Geometry: final body of the model. Coordinates: model frame, mm. Face numbers are marked on the shaded views. A direction names the side the tool comes from. Give positions to 0.01 mm unless a question says otherwise; leave off trailing zeros. Loops run counter-clockwise (first coordinate to the right, second up) from the corner with the lowest first, then second, coordinate; pieces in that order, holes last. Notation, with made-up numbers: (-9, 43.5) -> (42, 43.5) arc R23 ccw to (42, 74.5) -> close; hole circle Ø3 at (71, 87.25). An arc over 180 degrees is marked (long way). Answer in a Markdown table with one row per item. Add a question column.
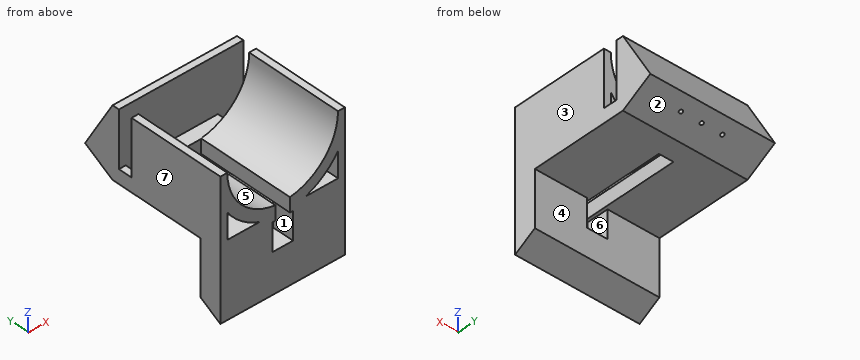
Autodesk Inventor part; units mm, degrees
ref_plane "YZ Plane" through (0, 0, 0) normal (1, 0, 0) x (0, 1, 0)
ref_plane "XZ Plane" through (0, 0, 0) normal (0, 1, 0) x (-1, 0, 0)
ref_plane "XY Plane" through (0, 0, 0) normal (0, 0, 1) x (1, 0, 0)
sketch "スケッチ1" plane through (0, 0, 0) normal (0, 1, 0) x (-1, 0, 0)
  line L0 (0, 0) -> (-90, 0)
  line L1 (-90, 0) -> (-90, 50)
  line L2 (0, 50) -> (0, 0)
  line L3 (0, 0) -> (-5, 0)
  line L4 (-5, 0) -> (-5, 50)
  line L5 (-5, 0) -> (-90, 0)
  line L6 (-90, 0) -> (-85, 0)
  line L7 (-85, 0) -> (-85, 50)
  arc A0 (-85, 50) -> (-5, 50) centre (-45, 50) ccw
  line L8 (0, 0) -> (0, 10)
  line L9 (0, 10) -> (-90, 10)
  circle A1 centre (-45, 50) radius 45
  line L10 (-90, 5) -> (0, 5)
  line L11 (-90, 50) -> (-85, 50)
  line L12 (-5, 50) -> (0, 50)
  line L13 (0, 0) -> (-90, 0)
  line L14 (-90, 0) -> (-90, 5)
  line L15 (-90, 5) -> (0, 5)
  line L16 (0, 5) -> (0, 0)
  dimension "d0" = 90
  dimension "d1" = 50
  dimension "d2" = 5
  dimension "d3" = 85
  dimension "d4" = 5
  dimension "d5" = 80
  dimension "d6" = 10
  dimension "d7" = 90
extrude "押し出し1" add sketch "スケッチ1" along normal blind 230 contours L0 L4 L10 L2 | L0 L7 L10 L4 | L10 L4 L9 L2 | L0 L1 L10 L7 | L10 A1 L9 L4 | L9 L4 A1 L2 | L10 L1 L9 L7 | L7 L9 A1 L10 | L9 A1 L4 | A1 L9 | A1 L4 L12 | L9 L1 A1 L7 | L7 A1 L9 | A1 L9 A0 L4 | A1 L7 A0 L9 | L11 L7 A1
sketch "スケッチ2" plane through (0, 0, 0) normal (0, -1, 0) x (1, 0, 0)
  line L0 (0, 0) -> (0, 50)
  line L1 (90, 0) -> (0, 0)
  line L2 (90, 50) -> (90, 0)
  line L3 (85, 50) -> (90, 50)
  arc A0 (5, 50) -> (85, 50) centre (45, 50) ccw
  line L4 (0, 50) -> (5, 50)
  arc A1 (5, 23.467) -> (85, 23.467) centre (45, 50) ccw
  line L5 (0, 5) -> (90, 5)
  line L6 (5, 23.467) -> (5, 5)
  line L7 (85, 23.467) -> (85, 5)
  dimension "d29" = 48
extrude "押し出し2" cut sketch "スケッチ2" against normal blind 225 contours L6 A1 L5 | L5 A1 L7
sketch "スケッチ3" plane through (0, 230, 0) normal (0, 1, 0) x (1, 0, 0)
  arc A0 (85, -50) -> (5, -50) centre (45, -50) ccw
  line L0 (90, -50) -> (90, 0)
  line L1 (0, -50) -> (5, -50)
  arc A1 (85, -50) -> (5, -50) centre (45, -50) ccw
  line L2 (5, -50) -> (85, -50)
extrude "押し出し3" add sketch "スケッチ3" against normal blind 5
sketch "スケッチ4" plane through (90, 0, 50) normal (1, 0, 0) x (0, 0, -1)
  line L0 (0, 0) -> (50, 0)
  line L1 (0, 0) -> (0, 230)
  line L2 (25, 0) -> (25, 65)
  line L3 (25, 65) -> (25, 75)
  line L4 (25, 75) -> (25, 215)
  line L5 (25, 215) -> (25, 225)
  line L6 (0, 65) -> (40, 65)
  line L7 (40, 65) -> (40, 75)
  line L8 (40, 75) -> (0, 75)
  line L9 (0, 75) -> (0, 65)
  line L10 (0, 215) -> (40, 215)
  line L11 (40, 215) -> (40, 225)
  line L12 (40, 225) -> (0, 225)
  line L13 (0, 225) -> (0, 215)
  dimension "d16" = 65
  dimension "d17" = 10
  dimension "d18" = 140
  dimension "d19" = 10
  dimension "d20" = 40
extrude "押し出し4" cut sketch "スケッチ4" against normal blind 90 contours L1 L8 L3 L6 | L3 L8 L7 L6 | L1 L12 L5 L10 | L5 L12 L11 L10
sketch "スケッチ6" plane through (90, 0, 50) normal (1, 0, 0) x (0, 0, -1)
  line L0 (0, 230) -> (50, 230)
  line L1 (50, 230) -> (37.5, 251.6506)
  line L2 (50, 230) -> (110, 230) construction
  line L3 (0, 230) -> (37.5, 251.6506)
  line L4 (0, 230) -> (43.3013, 230) construction
  dimension "d32" = 120
  dimension "d33" = 30
extrude "押し出し6" add sketch "スケッチ6" against normal blind 90
sketch "スケッチ9" plane through (0, 0, 0) normal (-1, 0, 0) x (0, 0, 1)
  line L0 (10, 225) -> (50, 225)
  line L1 (50, 225) -> (50, 230)
  line L2 (50, 230) -> (12.5, 251.6506)
  line L3 (12.5, 251.6506) -> (0, 230)
  line L4 (0, 0) -> (0, 230)
  line L5 (0, 0) -> (50, 0)
  line L6 (50, 0) -> (50, 65)
  line L7 (50, 65) -> (10, 65)
  line L8 (10, 65) -> (10, 75)
  line L9 (10, 75) -> (50, 75)
  line L10 (50, 75) -> (50, 215)
  line L11 (50, 215) -> (10, 215)
  line L12 (10, 215) -> (10, 225)
  line L13 (12.5, 251.6506) -> (0, 230)
  line L14 (0, 230) -> (-132.7906, 0)
  line L15 (0, 145) -> (-49.0748, 145)
  line L16 (0, 115) -> (-66.3953, 115)
  dimension "d45" = 30
sketch "スケッチ10" plane through (0, 0, 0) normal (-1, 0, 0) x (0, 0, 1)
  line L0 (10, 225) -> (50, 225)
  line L1 (50, 225) -> (50, 230)
  line L2 (50, 230) -> (12.5, 251.6506)
  line L3 (12.5, 251.6506) -> (0, 230)
  line L4 (0, 0) -> (0, 230)
  line L5 (0, 0) -> (50, 0)
  line L6 (50, 0) -> (50, 65)
  line L7 (50, 65) -> (10, 65)
  line L8 (10, 65) -> (10, 75)
  line L9 (10, 75) -> (50, 75)
  line L10 (50, 75) -> (50, 215)
  line L11 (50, 215) -> (10, 215)
  line L12 (10, 215) -> (10, 225)
  line L13 (12.5, 251.6506) -> (-87.5, 78.4456)
  line L14 (-87.5, 78.4456) -> (50, 0)
sketch "スケッチ11" plane through (90, 230, 0) normal (0, 0.5, -0.866) x (-1, 0, 0)
  line L0 (0, 25) -> (90, 25)
  line L1 (45, 25) -> (45, 15)
  line L2 (45, 15) -> (60, 15)
  line L3 (60, 15) -> (30, 15)
  point P0 (90, -199.1858)
  dimension "d49" = 10
  dimension "d50" = 15
  dimension "d51" = 30
hole "穴1" at (45, 242.9904, 7.5) at (30, 242.9904, 7.5) at (60, 242.9904, 7.5) direction (0, -0.5, 0.866) diameter 2.5 depth 8 tip angle 118
sketch "スケッチ18" plane through (90, 65, 10) normal (0, 0, 1) x (1, 0, 0)
  line L0 (0, 10) -> (-5, 10)
  line L1 (0, 10) -> (-90, 10)
  line L2 (-90, 10) -> (-90, 150)
  line L3 (-90, 150) -> (0, 150)
  line L4 (0, 150) -> (0, 10)
  line L5 (-45, 150) -> (-45, 10)
  line L6 (-53.1517, 150) -> (-27.646, 150)
  line L7 (-27.646, 150) -> (-27.646, 10)
  line L8 (-27.646, 10) -> (-53.1517, 10)
  line L9 (-53.1517, 10) -> (-53.1517, 150)
  line L10 (-45, 10) -> (-39.75, 10)
  line L11 (-45, 150) -> (-50.25, 150)
  line L12 (-50.25, 150) -> (-39.75, 150)
  line L13 (-39.75, 150) -> (-39.75, 10)
  line L14 (-39.75, 10) -> (-50.25, 10)
  line L15 (-50.25, 10) -> (-50.25, 150)
  point P0 (-90, -65)
  dimension "d76" = 140
  dimension "d77" = 5.25
  dimension "d78" = 5.25
extrude "押し出し12" cut sketch "スケッチ18" against normal blind 10 and the other way blind 5 contours L1 L5 L3 L13 | L1 L15 L3 L5
sketch "スケッチ19" plane through (0, 0, 0) normal (-1, 0, 0) x (0, 0, 1)
  line L0 (10, 225) -> (50, 225)
  line L1 (50, 225) -> (50, 230)
  line L2 (50, 230) -> (12.5, 251.6506)
  line L3 (12.5, 251.6506) -> (0, 230)
  line L4 (0, 0) -> (0, 230)
  line L5 (0, 0) -> (50, 0)
  line L6 (50, 0) -> (50, 65)
  line L7 (50, 65) -> (10, 65)
  line L8 (10, 65) -> (10, 75)
  line L9 (10, 75) -> (50, 75)
  line L10 (50, 75) -> (50, 215)
  line L11 (50, 215) -> (10, 215)
  line L12 (10, 215) -> (10, 225)
  line L13 (0, 230) -> (-23.825, 188.7339)
  line L14 (-23.825, 188.7339) -> (-3.4734, 176.9839)
  circle A0 centre (-3.4734, 176.9839) radius 16
  circle A1 centre (-3.4734, 176.9839) radius 3
  dimension "d83" = 47.65
  dimension "d84" = 23.5
  dimension "d85" = 32
  dimension "d86" = 6
sketch "スケッチ20" plane through (90, 230, 0) normal (0, 0.5, -0.866) x (-1, 0, 0)
  circle A0 centre (60, 15) radius 1.25
  circle A1 centre (45, 15) radius 1.25
  circle A2 centre (30, 15) radius 1.25
  line L0 (0, 0) -> (0, 25)
  line L1 (0, 0) -> (90, 0)
  line L2 (90, 25) -> (90, 0)
  line L3 (0, 25) -> (90, 25)
  point P0 (90, -199.1858)
ref_plane "作業平面5" through (90, 45, 50) normal (0, 1, 0) x (1, 0, 0)
sketch "スケッチ21" plane through (90, 45, 50) normal (0, 1, 0) x (1, 0, 0)
  line L0 (0, 0) -> (-101.8599, 0)
  line L1 (-101.8599, 0) -> (-101.8599, 60.1995)
  line L2 (-101.8599, 60.1995) -> (0, 60.1995)
  line L3 (0, 60.1995) -> (0, 0)
  point P0 (-90, 50)
extrude "押し出し13" cut sketch "スケッチ21" against normal blind 50
ref_plane "作業平面6" through (85, 145, 23.467) normal (0, 1, 0) x (-1, 0, 0)
sketch "スケッチ22" plane through (0, 75, 50) normal (-1, 0, 0) x (0, 0, 1)
  line L0 (-37.5, 176.6506) -> (-50, 155)
  line L1 (-50, -30) -> (-50, 155)
  line L2 (-98.8395, 70.6051) -> (-50, 70.6051)
  line L3 (-107.0544, 55.6051) -> (-50, 55.6051)
  line L4 (-89.7339, 85.6051) -> (-50, 85.6051)
  line L5 (-89.7339, 85.6051) -> (-107.0544, 55.6051)
  line L6 (-50, 55.6051) -> (-50, 85.6051)
  point P0 (-50, -75)
  dimension "d90" = 30
  dimension "d92" = 15
extrude "押し出し14" add sketch "スケッチ22" against normal blind 90
sketch "スケッチ23" plane through (0, 130.6051, -57.0544) normal (0, -1, 0) x (1, 0, 0)
  line L0 (0, 0) -> (90, 0)
  line L1 (39.75, 57.0544) -> (50.25, 57.0544)
  line L2 (45, 57.0544) -> (45, 0)
  line L3 (37.5, 57.0544) -> (52.5, 57.0544)
  line L4 (52.5, 57.0544) -> (52.5, 0)
  line L5 (52.5, 0) -> (37.5, 0)
  line L6 (37.5, 0) -> (37.5, 57.0544)
  line L7 (37.5, 57.0544) -> (52.5, 0) construction
  line L8 (52.5, 57.0544) -> (37.5, 0) construction
  line L9 (37.5, 57.0544) -> (52.5, 57.0544)
  line L10 (52.5, 57.0544) -> (52.5, 37.0544)
  line L11 (52.5, 37.0544) -> (37.5, 37.0544)
  line L12 (37.5, 37.0544) -> (37.5, 57.0544)
  point P0 (45, 28.5272)
  dimension "d95" = 15
  dimension "d96" = 20
extrude "押し出し15" cut sketch "スケッチ23" against normal blind 90 contours L6 L3 L1 L2 L11 | L2 L1 L3 L4 L11
sketch "スケッチ24" plane through (90, 230, 0) normal (0, 0, -1) x (-1, 0, 0)
  line L0 (50.25, -15) -> (50.25, -155)
  line L1 (50.25, -155) -> (39.75, -155)
  line L2 (39.75, -155) -> (39.75, -15)
  line L3 (39.75, -15) -> (50.25, -15)
  line L4 (52.5, -99.3949) -> (52.5, -69.3949)
  line L5 (52.5, -69.3949) -> (90, -69.3949)
  line L6 (90, -69.3949) -> (90, 0)
  line L7 (0, 0) -> (90, 0)
  line L8 (0, -69.3949) -> (0, 0)
  line L9 (0, -69.3949) -> (37.5, -69.3949)
  line L10 (37.5, -99.3949) -> (37.5, -69.3949)
  line L11 (37.5, -99.3949) -> (0, -99.3949)
  line L12 (0, -185) -> (0, -99.3949)
  line L13 (0, -185) -> (90, -185)
  line L14 (90, -185) -> (90, -99.3949)
  line L15 (90, -99.3949) -> (52.5, -99.3949)
  line L16 (0, -99.3949) -> (90, -99.3949)
  line L17 (90, -99.3949) -> (90, -69.3949)
  line L18 (90, -69.3949) -> (0, -69.3949)
  line L19 (0, -69.3949) -> (0, -99.3949)
  line L20 (-5, -64.3949) -> (95, -64.3949)
  line L21 (95, -64.3949) -> (95, -104.3949)
  line L22 (95, -104.3949) -> (-5, -104.3949)
  line L23 (-5, -104.3949) -> (-5, -64.3949)
  line L24 (-5, -64.3949) -> (95, -104.3949) construction
  line L25 (95, -64.3949) -> (-5, -104.3949) construction
  line L26 (0, -69.3949) -> (90, -69.3949)
  line L27 (90, -69.3949) -> (90, -99.3949)
  line L28 (90, -99.3949) -> (0, -99.3949)
  line L29 (0, -99.3949) -> (0, -69.3949)
  line L30 (0, -69.3949) -> (90, -99.3949) construction
  line L31 (90, -69.3949) -> (0, -99.3949) construction
  point P0 (90, -230)
  point P1 (45, -84.3949)
  dimension "d99" = 100
  dimension "d100" = 40
sketch "スケッチ25" plane through (90, 160.6051, -39.7339) normal (0, 0.5, -0.866) x (-1, 0, 0)
  line L0 (90, 0) -> (90, -34.641)
  line L1 (90, 0) -> (0, 0)
  line L2 (0, -34.641) -> (0, 0)
  line L3 (90, -34.641) -> (0, -34.641)
  point P0 (90, -119.2211)
sketch "スケッチ26" plane through (85, 145, 23.467) normal (0, 1, 0) x (-1, 0, 0)
  line L0 (125.1914, -92.9646) -> (-58.6843, -92.9646)
  line L1 (-58.6843, -92.9646) -> (-58.6843, 63.112)
  line L2 (-58.6843, 63.112) -> (125.1914, 63.112)
  line L3 (125.1914, 63.112) -> (125.1914, -92.9646)
  point P0 (85, -23.467)
extrude "押し出し16" cut sketch "スケッチ26" against normal blind 110
properties part number "知能ロボコン発射台２" material "ABS プラスチック"
(1) Cut plane D-D on y = 152.5. Return the cut outline in (x, z).
(2) Cut plane A-A on y = 183. Return the cut outline in (x, z).
(3) Draft query along X for the marked faces 1, 2 and 3. Return one class per face: +X half, -X half, draft (parallel to the pull), parting line (faces both ways), or undercut.
(4) Cut plane C-C on x = 83.5. Return the cut outline in (y, z).
(5) Material intervals for line 1 along X through (y, z) = (162, 8); line 2 along X through (y, z) = (194.5, 13.5); line 3 along X through (y, z) = (155.5, -3), sorted ascending. Write a range as from..to.
(6) Pin query (flat end, axial travel): pin 1 Ø12 at (x, z) = (12.5, 31) entering from +Y; pin 2 Ø8 at (x, y) = (46, 221.5) entering from +Z; pin 3 Ø1.5 at (x, y) = (77.5, 168.5) entering from +Z; pin 4 Ø6 at (x, y) = (71, 183) entering from -Z. Return the tip coordinate at first contact, or that it passes through.
(7) Reachability of the marked faces 4, 5, 6 and 7 from +Z, -Z, +X, -X, +Y, -Y: full face, straight path, thin tool, end or side. Return the list, or none.
(8) Cut plane B-B on z = -7.5. Return the cut outline in (x, y), then the cut area to 3 significant figures.
Answer list:
| question | item | result |
|---|---|---|
| 1 | outline | (0, -44.41) -> (90, -44.41) -> (90, 50) -> (85, 50) arc R40 cw to (50.25, 10.35) -> (50.25, 0) -> (52.5, 0) -> (52.5, -20) -> (37.5, -20) -> (37.5, 0) -> (39.75, 0) -> (39.75, 10.35) arc R40 cw to (5, 50) -> (0, 50) -> close; hole (5, 5) -> (28.3, 5) arc R48 cw to (5, 23.47) -> close; hole (61.7, 5) -> (85, 5) -> (85, 23.47) arc R48 cw to start |
| 2 | outline | (0, 0) -> (39.75, 0) -> (39.75, 10.35) arc R40 cw to (5, 50) -> (0, 50) -> close; (50.25, 0) -> (90, 0) -> (90, 50) -> (85, 50) arc R40 cw to (50.25, 10.35) -> close; hole (5, 5) -> (28.3, 5) arc R48 cw to (5, 23.47) -> close; hole (61.7, 5) -> (85, 5) -> (85, 23.47) arc R48 cw to start |
| 3 | face 1 | undercut |
| 3 | face 2 | draft |
| 3 | face 3 | +X half |
| 4 | outline | (145, -48.74) -> (160.61, -39.73) -> (160.61, 0) -> (230, 0) -> (251.65, 12.5) -> (230, 50) -> (225, 50) -> (225, 5) -> (145, 5) -> close; (145, 21.33) -> (215, 21.33) -> (215, 39.15) -> (145, 39.15) -> close |
| 5 | line 1 | x = 0..5, 21.76..39.75, 50.25..68.24, 85..90 |
| 5 | line 2 | x = 0..5, 13.83..28.64, 61.36..76.17, 85..90 |
| 5 | line 3 | x = 0..37.5, 52.5..90 |
| 6 | pin 1 | stops at y = 244.43 |
| 6 | pin 2 | stops at z = 50 |
| 6 | pin 3 | stops at z = 27.76 |
| 6 | pin 4 | stops at z = 0 |
| 7 | face 4 | -Z, +X, -X, +Y |
| 7 | face 5 | +Z, -Y |
| 7 | face 6 | +Y, -Y |
| 7 | face 7 | +Z, -Z, -X, +Y, -Y |
| 8 | outline | (0, 145) -> (37.5, 145) -> (37.5, 160.61) -> (0, 160.61) -> close; (52.5, 145) -> (90, 145) -> (90, 160.61) -> (52.5, 160.61) -> close |
| 8 | area | 1,170 mm² |
